Input: part model. Units: mm. Frame: model coordinates. Face numbers are marked on the shaded views. A direction names the side the tool comes from. Coordinates: 2 decimals unless noted, no trailing zeros. Write each loop counter-clockwise with the first axis right and the second up, starting at its lowest first coordinate (ties: lowest second). Pieces come first, ordered by that corner, then holes. Notation, with made-up numbers: (28.25, -6) - (49.25, -6) arc R34 ccw to (49.25, 24) - close; hole circle Ø5 at (-22.75, -14.75). An arc over 180 degrees is marked (long way). Use a Markdown table: item, result. Add a question column.
Q1. Pin query (flat end, axial travel): P1, Ø4, axis at x = 2.5, z = -4, coming from the +Y side; P2, Ø2.5, axis at x = 20.32, z = -3.175, coming from the +Y side; P3, Ø3, axis at y = 6, z = -20, coming from the +X side; P4, Ø5.5, axis at x = 20.5, z = -18.5, coming from the +Y side. Return the tip coordinate at first contact, or that it passes through.
Q2. Section query D-D (y = 4.75). Return the cut outline in (x, z), then the cut area to 3 significant figures.
Q3. Section query A-A (x = 20.32). Return the cut outline in (y, z) (3 decimals).
Q4. Mould query, pull axis Z, two halves, no side actions, for the marked faces 1, 2 and 3. Classes: released by +Z, released by -Z, zero draft, split by the parting line, or undercut.
Q5. Section query B-B (y = 11). Return the cut outline in (x, z) (3 decimals).
Q6. Material intervals for probe 1 along X at (y, z) = (9.25, -20.32); probe 2 along Z at (x, y) = (3.5, 11.75); probe 3 along Z at (x, y) = (20.32, 8), sorted ascending. Write a range as from..to.
Q7. Set-up query: the marked faces 4, 5, 6 and 7. Return all of +Z, -Z, +X, -X, +Y, -Y with unobstructed straight access to the full face (end or side cutting, diameter ignored); none if empty.
Q8. Section query C-C (z = -20.32). Return the cut outline in (x, y) (3 decimals).
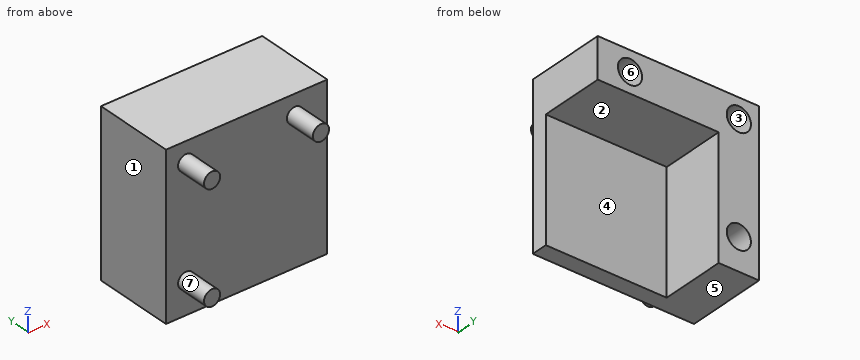
from build123d import *

# Parameters (mm, degrees)
SKETCH1_W           = 25.4
SKETCH1_H           = 25.4
BOSS_EXTRUDE1_DEPTH = 2.54
BOSS_EXTRUDE2_DEPTH = 10.16
SKETCH3_R           = 1.905
CUT_EXTRUDE1_DEPTH  = 6.35
SKETCH4_R           = 1.27
BOSS_EXTRUDE3_DEPTH = 5.08


with BuildPart() as part:
    # Sketch1 → Boss-Extrude1 (new body)
    with BuildSketch(Plane(origin=(0, 0, 0), x_dir=(1, 0, 0), z_dir=(0, 1, 0))):
        with Locations((12.7, 12.7)):
            Rectangle(SKETCH1_W, SKETCH1_H)
    extrude(amount=BOSS_EXTRUDE1_DEPTH)

    # Sketch2 → Boss-Extrude2 (add)
    with BuildSketch(Plane(origin=(0, 2.54, 0), x_dir=(1, 0, 0), z_dir=(0, 1, 0))):
        Polygon((0, 25.4), (0, 0), (25.4, 0), (25.4, 6.35), (6.35, 6.35), (6.35, 25.4), align=None)
    extrude(amount=BOSS_EXTRUDE2_DEPTH)

    # Sketch3 → Cut-Extrude1 (cut)
    with BuildSketch(Plane(origin=(0, 12.7, 0), x_dir=(1, 0, 0), z_dir=(0, 1, 0))):
        with Locations((3.175, 20.32)):
            Circle(SKETCH3_R)
        with Locations((3.175, 3.175)):
            Circle(SKETCH3_R)
        with Locations((20.32, 3.175)):
            Circle(SKETCH3_R)
    extrude(amount=-CUT_EXTRUDE1_DEPTH, mode=Mode.SUBTRACT)

    # Sketch4 → Boss-Extrude3 (add)
    with BuildSketch(Plane.XZ):
        with Locations((3.175, -3.175)):
            Circle(SKETCH4_R)
        with Locations((20.32, -3.175)):
            Circle(SKETCH4_R)
        with Locations((3.175, -20.32)):
            Circle(SKETCH4_R)
    extrude(amount=BOSS_EXTRUDE3_DEPTH)


solid = part.part
Values follow:
| question | item | result |
|---|---|---|
| 1 | P1 | y = 12.7 |
| 1 | P2 | y = 6.35 |
| 1 | P3 | x = 6.35 |
| 1 | P4 | y = 2.54 |
| 2 | outline | (0, -25.4) - (6.35, -25.4) - (6.35, -6.35) - (25.4, -6.35) - (25.4, 0) - (0, 0) - close |
| 2 | area | 282 mm2 |
| 3 | outline | (-5.08, -4.445) - (0, -4.445) - (0, -25.4) - (2.54, -25.4) - (2.54, -6.35) - (12.7, -6.35) - (12.7, -5.08) - (6.35, -5.08) - (6.35, -1.27) - (12.7, -1.27) - (12.7, 0) - (0, 0) - (0, -1.905) - (-5.08, -1.905) - close |
| 4 | face 1 | zero draft |
| 4 | face 2 | released by -Z |
| 4 | face 3 | undercut |
| 5 | outline | (0, -25.4) - (6.35, -25.4) - (6.35, -6.35) - (25.4, -6.35) - (25.4, 0) - (0, 0) - close; hole circle Ø3.81 at (3.175, -20.32); hole circle Ø3.81 at (3.175, -3.175); hole circle Ø3.81 at (20.32, -3.175) |
| 6 | probe 1 | 0..1.27, 5.08..6.35 |
| 6 | probe 2 | -25.4..-22.2, -18.44..-5.05, -1.3..0 |
| 6 | probe 3 | -6.35..-5.08, -1.27..0 |
| 7 | face 4 | -Z, +X, +Y |
| 7 | face 5 | -Z, +X, -X, +Y, -Y |
| 7 | face 6 | +Y |
| 7 | face 7 | -Y |
| 8 | outline | (0, 0) - (1.905, 0) - (1.905, -5.08) - (4.445, -5.08) - (4.445, 0) - (25.4, 0) - (25.4, 2.54) - (6.35, 2.54) - (6.35, 12.7) - (5.08, 12.7) - (5.08, 6.35) - (1.27, 6.35) - (1.27, 12.7) - (0, 12.7) - close |
